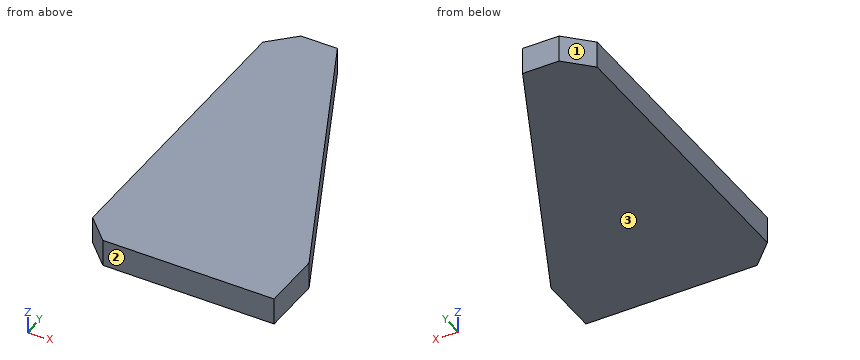
```python
from build123d import *

# Parameters (mm, degrees)
EXTRUDE_1_DEPTH = 20
CHAMFER_1_SIZE  = 18


with BuildPart() as part:
    # Эскиз1 → Бобышка-Вытянуть1 (new body)
    with BuildSketch(Plane.XY):
        Polygon((0, 0), (0, 45), (-100, 255), (-127, 255), (-145, 237), (-145, 0), align=None)
    extrude(amount=EXTRUDE_1_DEPTH)

    # Фаска1
    chamfer_1_edges = [part.edges().sort_by_distance(p)[0] for p in [
        (-145, 0, 10),
    ]]
    chamfer(chamfer_1_edges, length=CHAMFER_1_SIZE)


solid = part.part
```
Source: CAD feature listing. Evaluate the final solid. Frame: model axes, mm. Face numbers are marked on the shaded views. Give positions to 0.01 mm unless a question says otherwise; leave off trailing zeros. Write each loop counter-clockwise with the first axis right and the second up, starting at its lowest first coordinate (ties: lowest second). Pieces come first, ordered by that corner, then holes.
1. Pull-direction query (Y, two-part tool) for the marked faces 1, 2 and 3; classes: +Y half, -Y half, draft (parallel to the pull), parting line (faces both ways), or undercut.
2. Section query C-C (y = 168.5). Return the cut outline in (x, z).
3. Section query A-A (z = 7.5). Return the cut outline in (x, y), then the cut area to 3 significant figures.
4. Section query B-B (x = -15.5). Return the cut outline in (y, z), then the cut area to 3 significant figures.
5. First-contact query: pin 1 (2 mm diameter, centred on x = -62.5, z = 9.5, fed in from +Y); pin 2 (10 mm diameter, centred on y = 150.5, z = 12.5, fed in from +X). Flat tips, straight axial feed; report the tip coordinate or a pass-through.
6. Material intervals for line 1 along X through (y, z) = (94, 14.25); line 2 along X through (y, z) = (139.5, 1.75); line 3 along Y through (x, z) = (-80.5, 11), sorted ascending.
Output values:
1. face 1: +Y half
1. face 2: -Y half
1. face 3: draft
2. outline: (-145, 0) - (-58.81, 0) - (-58.81, 20) - (-145, 20) - close
3. outline: (-145, 18) - (-127, 0) - (0, 0) - (0, 45) - (-100, 255) - (-127, 255) - (-145, 237) - close
3. area: 26,200 mm2
4. outline: (0, 0) - (77.55, 0) - (77.55, 20) - (0, 20) - close
4. area: 1,550 mm2
5. pin 1: stops at y = 178.35
5. pin 2: stops at x = -47.86
6. line 1: x = -145 to -23.33
6. line 2: x = -145 to -45
6. line 3: y = 0 to 214.05
